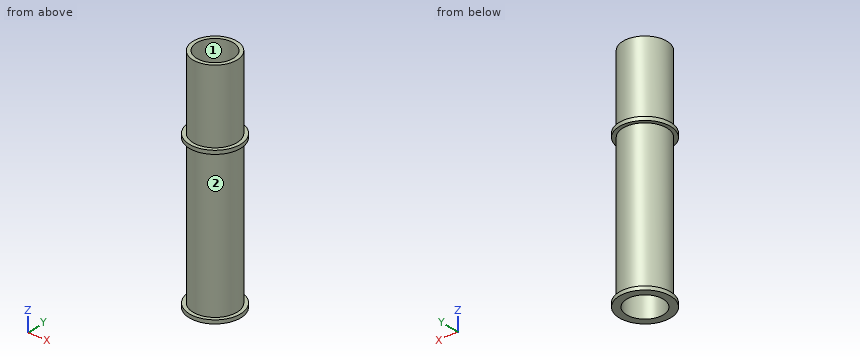
from build123d import *

# Parameters (mm, degrees)
SKETCH1_R           = 6
BOSS_EXTRUDE1_DEPTH = 40
SKETCH2_R           = 7
BOSS_EXTRUDE2_DEPTH = 1
BOSS_EXTRUDE3_START = 1
SKETCH3_R           = 7
BOSS_EXTRUDE3_DEPTH = 1
SKETCH4_R           = 6
BOSS_EXTRUDE4_DEPTH = 20
SKETCH5_R           = 5
CUT_EXTRUDE1_DEPTH  = 200


with BuildPart() as part:
    # Sketch1 → Boss-Extrude1 (new body)
    with BuildSketch(Plane.XY):
        Circle(SKETCH1_R)
    extrude(amount=BOSS_EXTRUDE1_DEPTH)

    # Sketch2 → Boss-Extrude2 (add)
    with BuildSketch(Plane(origin=(0, 0, 0), x_dir=(-1, 0, 0), z_dir=(0, 0, -1))):
        Circle(SKETCH2_R)
    extrude(amount=BOSS_EXTRUDE2_DEPTH)

    # Sketch3 → Boss-Extrude3 (add)
    with BuildSketch(Plane.XY.offset(40).offset(BOSS_EXTRUDE3_START)):
        with Locations(Location((0, 0, 0), (0, 0, 180))):
            Circle(SKETCH3_R)
    extrude(amount=-BOSS_EXTRUDE3_DEPTH)

    # Sketch4 → Boss-Extrude4 (add)
    with BuildSketch(Plane.XY.offset(41)):
        Circle(SKETCH4_R)
    extrude(amount=BOSS_EXTRUDE4_DEPTH)

    # Sketch5 → Cut-Extrude1 (cut)
    with BuildSketch(Plane.XY.offset(61)):
        Circle(SKETCH5_R)
    extrude(amount=-CUT_EXTRUDE1_DEPTH, mode=Mode.SUBTRACT)


solid = part.part
Verification items for the finished model (mm, model axes). Face numbers are marked on the shaded views. Give positions to 0.01 mm unless a question says otherwise; leave off trailing zeros. Order: outer loops, then holes, each group sorted by start corner. A loop starts at its lowest first (then second) coordinate and runs counter-clockwise, first axis right, second up. Notation, with made-up numbers: M -21,69.5 L -3,69.5 A21 ccw -3,79.5 Z; hole C -36,-36.75 d2. An arc over 180 degrees is marked long. Answer as a JSON object with one key per item and string values. Group by question number.
1) Depth check by flat-ended pin: pin 1 Ø4 at (x, y) = (1, 2.5) entering from +Z; pin 2 Ø8 at (x, z) = (1, 39.5) entering from +Y; pin 3 Ø1.5 at (x, z) = (3, 8.5) entering from -Y; pin 4 Ø2 at (x, z) = (2, 53) entering from +Y. Enter the tip coordinate at first touch or a pass-through.
2) Scan lines: line 1 along Y through (x, z) = (0, 37.5); line 2 along X through (y, z) = (0.5, 23); line 3 along X through (y, z) = (-2.25, 56). Record each from-to range of solid material in increasing order. Write a range as [from, to].
3) Cross-section at A-A (x = 0). Enter the section's corners in (y, z).
4) Mould release check, pull along Z, two halves, no side actions. Record for the marked faces 1 and 2: released by +Z, released by -Z, zero draft, split by the parting line, or undercut.
5) Cross-section at C-C (z = 5). Enter the section's corners in (x, y), then the cut area to 3 significant figures.
Result sheet:
{
 "1": {"pin 1": "passes through", "pin 2": "stops at y = 7", "pin 3": "stops at y = -5.56", "pin 4": "stops at y = 5.92"},
 "2": {"line 1": "y = [-6, -5], [5, 6]", "line 2": "x = [-5.98, -4.97], [4.97, 5.98]", "line 3": "x = [-5.56, -4.47], [4.47, 5.56]"},
 "3": {"outline": "M -7,-1 L -5,-1 L -5,61 L -6,61 L -6,41 L -7,41 L -7,40 L -6,40 L -6,0 L -7,0 Z; M 5,-1 L 7,-1 L 7,0 L 6,0 L 6,40 L 7,40 L 7,41 L 6,41 L 6,61 L 5,61 Z"},
 "4": {"face 1": "zero draft", "face 2": "undercut"},
 "5": {"outline": "C 0,0 d12; hole C 0,0 d10", "area": "34.6 mm2"}
}
